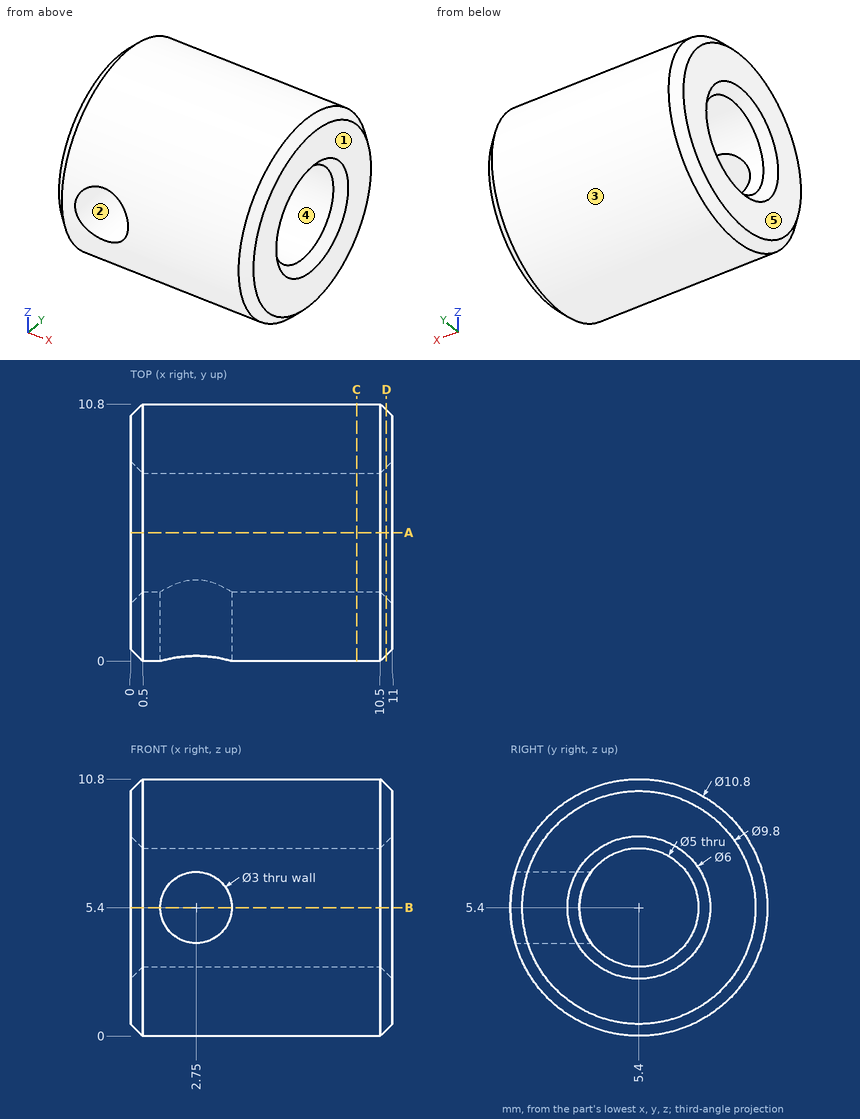
For this review, use the dimensioned drawing (mm, ordinates from the lowest corner) and the shaded views. A direction names the side the tool comes from. Give positions to 0.01 mm unless a question says otherwise; leave off trailing zeros. Order: outer loops, then holes, each group sorted by start corner. A loop starts at its lowest first (then second) coordinate and runs counter-clockwise, first axis right, second up.
1) The part is to be moulded in two halves that separate along Y. For the marked faces 3, 4 and 5, say which applies: released by +Y, released by -Y, zero draft, split by the parting line, or undercut.
2) Take a section at B-B (z = 5.4). Give the boundary of the cut face in (x, y).
3) Take a section at C-C (x = 9.5). Give the boundary of the cut face in (y, z), then the cut area to 3 significant figures.
4) Wall thickness on line 1 (Z direction, x = 7, y = 5.4); line 2 (Z direction, x = 6.5, y = 4); line 3 (Y direction, x = 7.5, z = 6): over which ranges is each line inside the solid? List them lowest first.
5) Take a section at A-A (y = 5.4). Give the boundary of the cut face in (x, z).
6) Insertion check: pin 1 (4 mm diameter, centred on x = 1, y = 9, fed in from -Z). The pin has a flat end and moves straight along its axis. Give the tip position at first contact, or say it passes through.
7) For the marked faces 1 and 2, list the 3-axis set-ups (+Z, -Z, +X, -X, +Y, -Y) from which the entire face can be reached by the end or side of a thin tool; tool diameter is ignored.
8) Take a section at D-D (x = 10.75). Give the boundary of the cut face in (y, z), then the cut area to 3 significant figures.
Derived:
1. face 3: split by the parting line
1. face 4: undercut
1. face 5: zero draft
2. outline: (0, 0.5) - (0.5, 0) - (1.25, 0) - (1.25, 2.9) - (0.5, 2.9) - (0, 2.4) - close; (0, 8.4) - (0.5, 7.9) - (10.5, 7.9) - (11, 8.4) - (11, 10.3) - (10.5, 10.8) - (0.5, 10.8) - (0, 10.3) - close; (4.25, 0) - (10.5, 0) - (11, 0.5) - (11, 2.4) - (10.5, 2.9) - (4.25, 2.9) - close
3. outline: circle Ø10.8 at (5.4, 5.4); hole circle Ø5 at (5.4, 5.4)
3. area: 72.0 mm2
4. line 1: z = 0 to 2.9, 7.9 to 10.8
4. line 2: z = 0.18 to 3.33, 7.47 to 10.62
4. line 3: y = 0.03 to 2.97, 7.83 to 10.77
5. outline: (0, 0.5) - (0.5, 0) - (10.5, 0) - (11, 0.5) - (11, 2.4) - (10.5, 2.9) - (0.5, 2.9) - (0, 2.4) - close; (0, 8.4) - (0.5, 7.9) - (10.5, 7.9) - (11, 8.4) - (11, 10.3) - (10.5, 10.8) - (0.5, 10.8) - (0, 10.3) - close
6. pin 1: stops at z = 0.24
7. face 1: +Z, -Z, +X, +Y, -Y
7. face 2: -Y
8. outline: circle Ø10.3 at (5.4, 5.4); hole circle Ø5.5 at (5.4, 5.4)
8. area: 59.6 mm2
